Autodesk Inventor part; units mm, degrees
ref_plane "YZ Plane" through (0, 0, 0) normal (1, 0, 0) x (0, 1, 0)
ref_plane "XZ Plane" through (0, 0, 0) normal (0, 1, 0) x (-1, 0, 0)
ref_plane "XY Plane" through (0, 0, 0) normal (0, 0, 1) x (1, 0, 0)
sketch "Sketch1" plane through (0, 0, 0) normal (0, 0, 1) x (1, 0, 0)
  line L0 (0, 0) -> (6, 0)
  line L1 (6, 0) -> (6, 11)
  line L2 (0, 0) -> (0, 15)
  line L3 (0, 15) -> (2, 15)
  line L4 (2, 15) -> (6, 11)
  dimension "d0" = 6
  dimension "d1" = 11
  dimension "d2" = 15
  dimension "d3" = 2
extrude "Extrusion1" add sketch "Sketch1" along normal blind 96
sketch "Sketch2" plane through (0, 0, 0) normal (0, -1, 0) x (1, 0, 0)
  line L0 (0, 0) -> (0, 96)
  line L1 (5.9866, 0) -> (0, 0)
  line L2 (0, 96) -> (6, 96)
  line L3 (0, 96) -> (6, 96)
  line L4 (6, 96) -> (6, 90)
  line L5 (6, 90) -> (0, 96)
  line L6 (0, 0) -> (6, 0)
  line L7 (6, 0) -> (0, 0)
  line L8 (6, 0) -> (6, 6)
  line L9 (6, 0) -> (6, 96)
  line L10 (6, 6) -> (0, 0)
  dimension "d7" = 6
  dimension "d8" = 6
extrude "Extrusion2" cut sketch "Sketch2" against normal blind 42.1125 contours L10 L8 L6 L1 | L2 L4 L5
sketch "Sketch3" plane through (6, 0, 90) normal (1, 0, 0) x (0, 0, -1)
  line L0 (84, 11) -> (0, 11)
  line L1 (84, 0) -> (0, 0)
  line L2 (42, 11) -> (42, 0)
  line L3 (42, 0) -> (48, 0)
  line L4 (90, 0) -> (-6, 0)
  line L5 (48, 0) -> (48, 11)
  line L6 (42, 0) -> (36, 0)
  line L7 (36, 0) -> (36, 11)
  line L8 (42, 11) -> (42, 15)
  line L9 (88, 15) -> (-4, 15)
  line L10 (42, 15) -> (44, 15)
  line L11 (44, 15) -> (48, 11)
  line L12 (42, 15) -> (40, 15)
  line L13 (40, 15) -> (36, 11)
  point P0 (36, 0)
  dimension "d11" = 6
  dimension "d12" = 6
  dimension "d13" = 2
  dimension "d14" = 2
extrude "Extrusion3" add sketch "Sketch3" against normal blind 6
sketch "Sketch4" plane through (6, 0, 90) normal (1, 0, 0) x (0, 0, -1)
  line L0 (36, 11) -> (0, 11)
  line L1 (0, 11) -> (0, 0)
  line L2 (84, 0) -> (0, 0)
  line L3 (84, 0) -> (84, 11)
  line L4 (84, 11) -> (48, 11)
  line L5 (48, 11) -> (44, 15)
  line L6 (44, 15) -> (40, 15)
  line L7 (40, 15) -> (36, 11)
  line L8 (84, 0) -> (0, 0)
  line L9 (42, 0) -> (42, 7.5)
  circle A0 centre (42, 7.5) radius 3.2
  point P0 (90, 0)
  dimension "d17" = 7.5
  dimension "d18" = 6.4
extrude "Extrusion4" cut sketch "Sketch4" against normal blind 10 contours A0
properties part number "edge-join-hole"
Input: part model. Units: mm. Frame: model coordinates. A direction names the side the tool comes from. Coordinates: 2 decimals unless noted, no trailing zeros. Order: outer loops, then holes, each group sorted by start corner. A loop starts at its lowest first (then second) coordinate and runs counter-clockwise, first axis right, second up. Notation, with made-up numbers: M 35,-39.5 L 85,-39.5 A13 ccw 85,-25.5 Z; hole C 31,-10 d3. An arc over 180 degrees is marked long. Write item = value, one per line. Start each with the question number.
(1) Pull-direction query (Y, two-part tool) for faces 4 (the cylindrical face through (3.042, 4.661, 46.523)), 5 (the flat face through (4, 13, 24)), 6 (the flat face through (3, 7, 93)); classes: released by +Y, released by -Y, zero draft, split by the parting line, or undercut.
(2) Section D-D on y = 14. Output: boundary loops of the cut face in (x, z), and give its area (3 significant figures).
(3) Section C-C on x = 3. Output: boundary loops of the cut face in (y, z), and give its area (3 significant figures).
(4) Section A-A on z = 48. Output: boundary loops of the cut face in (x, y).
(5) Reachability of faces 1 (the flat face through (4.5, 13.5, 44.5)), 2 (the flat face through (0, 4, 47)), 3 (the flat face through (4.5, 13.5, 51.5)) from +Z, -Z, +X, -X, +Y, -Y: full face, straight path, thin tool, end or side. Return the list, or none.
(6) Line query: line 1 along Y through (x, z) = (3.5, 48); line 2 along Z through (x, y) = (4, 10.25); line 3 along Y through (x, z) = (4, 50.5). Output: solid intervals per line, ascending. Write a range as [from, to].
(7) Section B-B on y = 7.5. Output: boundary loops of the cut face in (x, z), and give its area (3 significant figures).
(8) First-contact query: P1, Ø3, axis at x = 4.5, y = 2, coming from the -Z side; P2, Ø1, axis at x = 4.5, y = 11.5, coming from the +Z side; P3, Ø1.5, axis at x = 2.5, y = 12, coming from the -Z side. Flat tips, straight axial feed; report the tip coordinate or a pass-through.
Result set:
q1.face_4 = undercut
q1.face_5 = released by +Y
q1.face_6 = zero draft
q2.outline = M 0,0 L 3,3 L 3,45 L 6,45 L 6,51 L 3,51 L 3,93 L 0,96 Z
q2.area = 297 mm²
q3.outline = M 0,3 L 14,3 L 14,45 L 15,46 L 15,50 L 14,51 L 14,93 L 0,93 Z; hole C 7.5,48 d6.4
q3.area = 1,230 mm²
q4.outline = M 0,0 L 6,0 L 6,4.3 L 0,4.3 Z; M 0,10.7 L 6,10.7 L 6,15 L 0,15 Z
q5.face_1 = -Z, +X, +Y
q5.face_2 = +Z, -Z, -X, +Y, -Y
q5.face_3 = +Z, +X, +Y
q6.line_1 = [0, 4.3], [10.7, 15]
q6.line_2 = [4, 46.36], [49.64, 92]
q6.line_3 = [0, 5.5], [9.5, 14.5]
q7.outline = M 0,0 L 6,6 L 6,44.8 L 0,44.8 Z; M 0,51.2 L 6,51.2 L 6,90 L 0,96 Z
q7.area = 502 mm²
q8.P1 = 3
q8.P2 = 92
q8.P3 = 1.75
